Autodesk Inventor part; units mm, degrees
ref_plane "YZ Plane" through (0, 0, 0) normal (1, 0, 0) x (0, 1, 0)
ref_plane "XZ Plane" through (0, 0, 0) normal (0, 1, 0) x (-1, 0, 0)
ref_plane "XY Plane" through (0, 0, 0) normal (0, 0, 1) x (1, 0, 0)
sketch "Sketch1" plane through (0, 0, 0) normal (1, 0, 0) x (0, 1, 0)
  line L0 (0, 0) -> (50.8, 0)
  line L1 (50.8, 0) -> (50.8, -25.4)
  line L2 (50.8, -25.4) -> (0, -25.4)
  line L3 (0, -25.4) -> (0, 0)
  line L4 (49.53, -24.13) -> (49.53, -1.27)
  line L5 (49.53, -1.27) -> (1.27, -1.27)
  line L6 (1.27, -1.27) -> (1.27, -24.13)
  line L7 (1.27, -24.13) -> (49.53, -24.13)
  dimension "d0" = 50.8
  dimension "d1" = 25.4
  dimension "d2" = 1.27
extrude "Extrusion1" add sketch "Sketch1" along normal blind 609.6
sketch "Sketch2" plane through (0, 0, 0) normal (0, 0, 1) x (1, 0, 0)
  line L0 (537.5598, 19.0095) -> (541.0559, 18.8772)
  line L1 (534.0637, 19.1419) -> (537.5598, 19.0095)
  line L2 (532.1846, 22.3903) -> (533.818, 19.2964)
  arc A0 (533.818, 19.2964) -> (534.0637, 19.1419) centre (537.8, 25.355) ccw
  arc A1 (530.5621, 25.7742) -> (530.5512, 25.4841) centre (537.8, 25.355) ccw
  arc A2 (534.5441, 31.8328) -> (534.2874, 31.6973) centre (537.8, 25.355) ccw
  arc A3 (541.782, 31.4136) -> (541.5363, 31.5681) centre (537.8, 25.355) ccw
  arc A4 (545.0379, 24.9358) -> (545.0488, 25.2259) centre (537.8, 25.355) ccw
  arc A5 (541.0559, 18.8772) -> (541.3126, 19.0127) centre (537.8, 25.355) ccw
  circle A6 centre (537.8, 25.355) radius 7.25
  point P0 (0, 0)
extrude "Extrusion2" cut sketch "Sketch2" against normal through all
sketch "Sketch4" plane through (0, 0, 0) normal (0, 0, 1) x (1, 0, 0)
  circle A0 centre (352.9118, 25.4) radius 7.3323
  circle A1 centre (174.2245, 25.4) radius 7.3323
  point P0 (0, 0)
extrude "Extrusion4" cut sketch "Sketch4" against normal through all
properties part number "Aluminum Channel Arm"
Can you work these out from the model? Positions are in its coordinate system, mm. A direction names the side the tool comes from. Coordinates: 2 decimals unless noted, no trailing zeros. Write each loop counter-clockwise with the first axis right and the second up, starting at its lowest first coordinate (ties: lowest second). Pieces come first, ordered by that corner, then holes. Notation, with made-up numbers: (76.5, 5) -> (116.5, 5) arc R22 ccw to (116.5, 40) -> close; hole circle Ø5 at (-22.5, 60). An arc over 180 degrees is marked (long way). Answer as CSV lines item,"result".
1) On a 3-axis mill with a long thin cutter (end or side, diameter ignored), from which of +Z, -Z, +X, -X, +Y, -Y can I reach the whole of each face in a straight line? I mean faces 1 (the cylindrical face through (181.22, 27.6, -0.63)), 2 (the flat face through (301, 25, -24.13)). Say none if no direction works.
Check result:
face 1,"+Z, -Z"
face 2,"+X, -X"
2) If we section it at A-A on x = 390.5: Please give me the cut outline in (y, z), then the cut area to 3 significant figures.
Check result:
outline,"(0, -25.4) -> (50.8, -25.4) -> (50.8, 0) -> (0, 0) -> close; hole (1.27, -24.13) -> (49.53, -24.13) -> (49.53, -1.27) -> (1.27, -1.27) -> close"
area,"187 mm²"
3) If we section it at B-B on z = -12.5: Please give me the cut outline in (x, y), then the cut area to 3 significant figures.
Check result:
outline,"(0, 0) -> (609.6, 0) -> (609.6, 1.27) -> (0, 1.27) -> close; (0, 49.53) -> (609.6, 49.53) -> (609.6, 50.8) -> (0, 50.8) -> close"
area,"1,550 mm²"
4) If I drill on line 1 (Y direction, x = 121, z = -1.5); line 2 (Z direction, x = 156.5, y = 32), over which ranges is the centre line in solid material (lowest first)? Write a range as from..to.
Check result:
line 1,"0..1.27, 49.53..50.8"
line 2,"-25.4..-24.13, -1.27..0"
5) If we mould it in two halves opening along Y, with no side actions, what happens to faces 3 (the cylindrical face through (359.685, 22.592, -0.626)), 4 (the flat face through (301, 0, -13)), 5 (the flat face through (301, 50.8, -13)), 6 (the flat face through (301, 26, -25.4))? For each: +Y half, -Y half, draft (parallel to the pull), parting line (faces both ways), or undercut.
Check result:
face 3,"undercut"
face 4,"-Y half"
face 5,"+Y half"
face 6,"draft"
